Here's how the part is built. I have some questions about the finished solid (model axes, mm). Give positions to 0.01 mm unless a question says otherwise; leave off trailing zeros. Write each loop counter-clockwise with the first axis right and the second up, starting at its lowest first coordinate (ties: lowest second). Pieces come first, ordered by that corner, then holes. Notation, with made-up numbers: (68, -2.75) - (78, -2.75) arc R28 cw to (78, 32.25) - close; hole circle Ø2 at (49.25, -28). An arc over 180 degrees is marked (long way). One line per item, written item: value. Start each with the question number.
1) Please list where these lines run through material, in increasing order: L1, parallel to Y at x = 0, z = 0.6; L2, parallel to X at y = 10.5, z = 1.6; L3, parallel to Y at x = -40.5, z = 1.7. Write a range as [from, to].
2) I'm going to push flat-ended pins straight in: P1, Ø2, axis at x = 29.5, y = -27, coming from the -Z side; P2, Ø2.5, axis at x = -29.77, y = -29.77, coming from the +Z side. Where does each tip first touch, or does it pass through?
3) Imagine slicing it at A-A on y = 0. Write out the boundary of the cut face in (x, z), plus the area to 3 significant figures.
4) Imagine slicing it at D-D on z = 0.5. Write out the boundary of the cut face in (x, y), plus the area to 3 significant figures.
5) Imagine slicing it at C-C on x = -10.5. Write out the boundary of the cut face in (y, z), plus the area to 3 significant figures.
6) We'd pull the mould along Y, two halves only. Please class faces 1 (the cylindrical face through (-9.237, 40.297, 1.014)), 2 (the cylindrical face through (-39.52, 12.15, 1.01)), 3 (the flat face through (-17.33, -34.01, 2)), 4 (the cylindrical face through (-10.02, 45.1, 0.99)): +Y half, -Y half, draft (parallel to the pull), parting line (faces both ways), or undercut.
Solid Edge part; units mm, degrees
sketch "Sketch1" plane through (0, 0, 0) normal (0, 0, 1) x (1, 0, 0)
  circle A0 centre (0, 0) radius 38
  circle A1 centre (0, 0) radius 46.2
extrude "Protrusion1" add sketch "Sketch1" along normal blind 2
hole "Hole1" at (29.7692, 29.7692, 2) direction (0, 0, -1) diameter 3.4 end up to next
pattern_circular "Pattern1" count 6 over 360 about axis through (0, 0, 2) along (0, 0, -1) of "Hole1"
Numbers:
1. L1: [-46.2, -38], [38, 46.2]
1. L2: [-44.99, -42.32], [-39.01, -36.52], [36.52, 44.99]
1. L3: [-22.23, 9.2], [12.59, 22.23]
2. P1: z = 0
2. P2: through
3. outline: (-46.2, 0) - (-38, 0) - (-38, 2) - (-46.2, 2) - close; (38, 0) - (46.2, 0) - (46.2, 2) - (38, 2) - close
3. area: 32.8 mm^2
4. outline: circle Ø92.4 at (0, 0); hole circle Ø3.4 at (-40.67, 10.9); hole circle Ø76 at (0, 0); hole circle Ø3.4 at (-29.77, -29.77); hole circle Ø3.4 at (-10.9, 40.67); hole circle Ø3.4 at (10.9, -40.67); hole circle Ø3.4 at (29.77, 29.77); hole circle Ø3.4 at (40.67, -10.9)
4. area: 2,110 mm^2
5. outline: (-44.99, 0) - (-36.52, 0) - (-36.52, 2) - (-44.99, 2) - close; (36.52, 0) - (39.01, 0) - (39.01, 2) - (36.52, 2) - close; (42.32, 0) - (44.99, 0) - (44.99, 2) - (42.32, 2) - close
5. area: 27.3 mm^2
6. face 1: undercut
6. face 2: undercut
6. face 3: draft
6. face 4: parting line
